Could you check a few things on this model? Use its own coordinates, in mm. A direction names the side the tool comes from. Coordinates: 2 decimals unless noted, no trailing zeros. Order: outer loops, then holes, each group sorted by start corner. A loop starts at its lowest first (then second) coordinate and runs counter-clockwise, first axis right, second up. Notation, with made-up numbers: (-2, 61) - (34, 61) arc R19 cw to (34, 70) - close; hole circle Ø4 at (-1.5, 45). An arc over 180 degrees is marked (long way). One line per item, written item: value.
from build123d import *

# Parameters (mm, degrees)
F0_W     = 28.933504
F0_H     = 151.753276
F1_DEPTH = 15.24
F2_W     = 2.633254
F2_H     = 23.030557
F3_DEPTH = 2.54


with BuildPart() as f1:
    # F0 (on Top) → F1 (new body)
    with BuildSketch(Plane.XY):
        Rectangle(F0_W, F0_H)
    extrude(amount=F1_DEPTH)

    # F2 (on face) → F3 (cut)
    with BuildSketch(Plane.XY.offset(15.24)):
        Polygon((-4.133359, 47.533616), (4.133359, 47.533616), (4.368631, 47.533616), (0, 55.100307), (-4.368631, 47.533616), align=None)
        Polygon((4.133359, -47.533616), (4.133359, 47.533616), (-4.133359, 47.533616), (-4.133359, -47.533616), (-1.316627, -47.533616), (1.316627, -47.533616), align=None)
        with Locations((0, -59.048894)):
            Rectangle(F2_W, F2_H)
    extrude(amount=-F3_DEPTH, mode=Mode.SUBTRACT)


solid = f1.part
Item 1: I want a section at B-B on y = -65. Please give me the cut outline in (x, z), then the cut area to 3 significant figures.
Conclusion:
outline: (-14.47, 0) - (14.47, 0) - (14.47, 15.24) - (1.32, 15.24) - (1.32, 12.7) - (-1.32, 12.7) - (-1.32, 15.24) - (-14.47, 15.24) - close
area: 434 mm²
Item 2: I want a section at A-A on y = -3. Please give me the cut outline in (x, z), then the cut area to 3 significant figures.
Conclusion:
outline: (-14.47, 0) - (14.47, 0) - (14.47, 15.24) - (4.13, 15.24) - (4.13, 12.7) - (-4.13, 12.7) - (-4.13, 15.24) - (-14.47, 15.24) - close
area: 420 mm²
Item 3: Thinking about a two-plate mould opening in Y: for faces 1 (the face through (0, 1, 0)), 2 (the face through (0, 75.877, 8)), 3 (the face through (3, -47.534, 14)), which applies, pulls with the +Y half, pulls with the -Y half, needs draft (parallel to the pull), parting line crosses it, or undercut?
Conclusion:
face 1: needs draft
face 2: pulls with the +Y half
face 3: undercut
Item 4: If I drill on probe 1 along X at (y, z) = (-27.5, 14.25); probe 2 along Z at (x, y) = (1.75, 0); probe 3 along Y at (x, z) = (-2, 14.5), over which ranges is the centre line in solid material (lowest first)?
Conclusion:
probe 1: -14.47 to -4.13, 4.13 to 14.47
probe 2: 0 to 12.7
probe 3: -75.88 to -47.53, 51.64 to 75.88
Item 5: For faces 4 (the face through (0, -75.877, 8)), 5 (the face through (1.317, -59, 14)), which set-ups out of +Z, -Z, +X, -X, +Y, -Y let a thin tool reach every point of the face, with its end or its side?
Conclusion:
face 4: +Z, -Z, +X, -X, -Y
face 5: +Z
